Autodesk Inventor part; units mm, degrees
ref_plane "YZ Plane" through (0, 0, 0) normal (1, 0, 0) x (0, 1, 0)
ref_plane "XZ Plane" through (0, 0, 0) normal (0, 1, 0) x (-1, 0, 0)
ref_plane "XY Plane" through (0, 0, 0) normal (0, 0, 1) x (1, 0, 0)
sketch "Boceto1" plane through (0, 0, 0) normal (0, 0, 1) x (1, 0, 0)
  circle A0 centre (0, 0) radius 13.175
  circle A1 centre (0, 0) radius 11.5
  dimension "d0" = 26.35
  dimension "d1" = 23
extrude "Extrusión1" add sketch "Boceto1" along normal blind 130
sketch "Boceto2" plane through (0, 0, 0) normal (1, 0, 0) x (0, 1, 0)
  line L0 (1.5, 5) -> (1.5, 0)
  line L1 (-13.175, 0) -> (13.175, 0)
  line L2 (1.5, 0) -> (-1.5, 0)
  line L3 (-1.5, 0) -> (-1.5, 5)
  line L4 (1.5, 5) -> (-1.5, 5)
  point P0 (0, 0)
  dimension "d6" = 3
extrude "Extrusión2" cut sketch "Boceto2" along normal mid plane 130
sketch "Boceto3" plane through (0, 0, 0) normal (1, 0, 0) x (0, 1, 0)
  line L0 (13.175, 130) -> (-13.175, 130)
  line L1 (1.5, 130) -> (-1.5, 130)
  line L2 (1.5, 130) -> (1.5, 120)
  line L3 (1.5, 120) -> (-1.5, 120)
  line L4 (-1.5, 120) -> (-1.5, 130)
  point P0 (0, 0)
  dimension "d10" = 3
  dimension "d11" = 10
  dimension "d12" = 3
extrude "Extrusión3" cut sketch "Boceto3" along normal mid plane 30
properties part number "tubo"
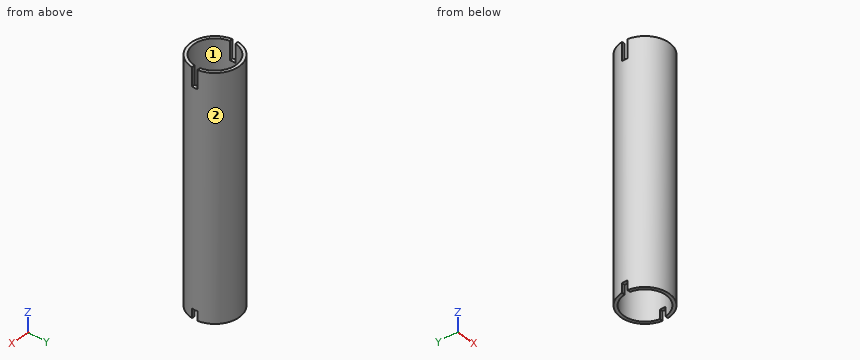
Design review of the part built by this model. Coordinates are the model's own, in mm. Face numbers are marked on the shaded views. Coordinates: 2 decimals unless noted, no trailing zeros. Order: outer loops, then holes, each group sorted by start corner. A loop starts at its lowest first (then second) coordinate and runs counter-clockwise, first axis right, second up. Notation, with made-up numbers: (57.5, -25.75) -> (79.5, -25.75) arc R24 cw to (79.5, -12.75) -> close; hole circle Ø3 at (-17.75, 70.25). An arc over 180 degrees is marked (long way). One line per item, written item: value. Start each with the question number.
Q1. Mouldability with a two-part tool opening along X and no side actions: class the marked faces 1 and 2 as pulls with the +X half, pulls with the -X half, needs draft (parallel to the pull), parting line crosses it, or undercut.
Q2. Insertion check: pin 1 Ø0.8 at (x, z) = (-12, 1.5) entering from -Y; pin 2 Ø0.5 at (x, y) = (12, 0) entering from +Z; pin 3 Ø1.4 at (x, z) = (12, 124.5) entering from +Y; pin 4 Ø12 at (x, y) = (-1, -7) entering from +Z. Each pin has a flat end and moves straight along its axis. Give the tip position at first contact, or say it passes through.
Q3. Take a section at C-C, the plane z = 66.5. State the section outline as (x, y) points (3 decimals).
Q4. For probe 1 along X at (y, z) = (-8.5, 64); probe 2 along Y at (x, z) = (1, 41); probe 3 along X at (y, z) = (-0.75, 6), list the stretches that pass through material, from the lowest coordinate up.
Q5. Take a section at B-B, the plane x = 0. State the section outline as (y, z) points (3 decimals).
Q6. Take a section at A-A, the plane y = 0. State the section outline as (x, z) points (3 decimals).
Values follow:
1. face 1: undercut
1. face 2: parting line crosses it
2. pin 1: stops at y = -6.25
2. pin 2: stops at z = 120
2. pin 3: stops at y = 6.77
2. pin 4: stops at z = 130
3. outline: circle Ø26.35 at (0, 0); hole circle Ø23 at (0, 0)
4. probe 1: x = -10.07 to -7.75, 7.75 to 10.07
4. probe 2: y = -13.14 to -11.46, 11.46 to 13.14
4. probe 3: x = -13.15 to -11.48, 11.48 to 13.15
5. outline: (-13.175, 0) -> (-11.5, 0) -> (-11.5, 130) -> (-13.175, 130) -> close; (11.5, 0) -> (13.175, 0) -> (13.175, 130) -> (11.5, 130) -> close
6. outline: (-13.175, 5) -> (-11.5, 5) -> (-11.5, 120) -> (-13.175, 120) -> close; (11.5, 5) -> (13.175, 5) -> (13.175, 120) -> (11.5, 120) -> close
